For this review, take the finished solid that the model builds, in its own axes (mm). Coordinates: 2 decimals unless noted, no trailing zeros. Loops run counter-clockwise (first coordinate to the right, second up) from the corner with the lowest first, then second, coordinate; pieces in that order, holes last. Notation, with made-up numbers: M 3,21 L 27,21 A14 cw 27,34 Z; hole C 38,-33.75 d11. An arc over 180 degrees is marked long. Answer as a JSON object with one key per item and string values. Group by question number.
Item 1: Insertion check: pin 1 (10 mm diameter, centred on x = -296.88, z = -246.55, fed in from -Y); pin 2 (4 mm diameter, centred on x = -177.8, z = -40.3, fed in from -Y). Each pin has a flat end and moves straight along its axis. Give the tip position at first contact, or say it passes through.
Item 2: Add section A-A (z = -177.8). State the section outline as (x, y) points (3 decimals), then the cut area to 3 significant figures.
Item 3: Add section C-C (y = 1.6). Count the separate pieces of the cut face and the enclosed holes in it, then the cut area to 3 significant figures.
Item 4: Add section B-B (x = -191). State the section outline as (y, z) points (3 decimals), then the cut area to 3 significant figures.
Item 5: Wall thickness on L1, parallel to Z at x = -177.8, y = 1.95 (3 decimals); L2, parallel to X at y = 2.65, z = -316; L3, parallel to X at y = 1.7, z = -246.55: over which ranges is each line inside the solid? List them lowest first. Write a range as from..to.
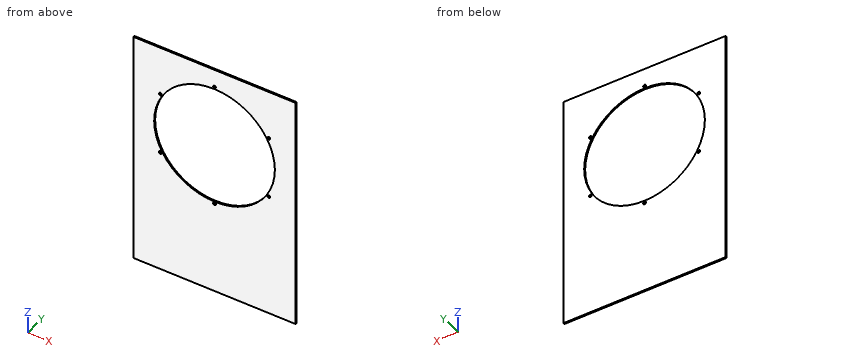
Autodesk Inventor part; units mm, degrees
ref_plane "YZ Plane" through (0, 0, 0) normal (1, 0, 0) x (0, 1, 0)
ref_plane "XZ Plane" through (0, 0, 0) normal (0, 1, 0) x (-1, 0, 0)
ref_plane "XY Plane" through (0, 0, 0) normal (0, 0, 1) x (1, 0, 0)
sketch "Sketch1" plane through (0, 0, 0) normal (0, 1, 0) x (-1, 0, 0)
  line L0 (0, 0) -> (355.6, 0)
  line L1 (355.6, 0) -> (355.6, -520.7)
  line L2 (355.6, -520.7) -> (0, -520.7)
  line L3 (0, -520.7) -> (0, 0)
  circle A0 centre (177.8, -177.8) radius 132.516
  circle A1 centre (177.8, -315.3) radius 3.175
  circle A2 centre (296.8785, -246.55) radius 3.175
  circle A3 centre (296.8785, -109.05) radius 3.175
  circle A4 centre (177.8, -40.3) radius 3.175
  circle A5 centre (58.7215, -109.05) radius 3.175
  circle A6 centre (58.7215, -246.55) radius 3.175
  line L4 (177.8, -177.8) -> (330.2, -177.8) construction
  line L5 (177.8, -177.8) -> (309.7823, -254) construction
  point P0 (177.8, -520.7)
  point P1 (355.6, -260.35)
  dimension "d0" = 355.6
  dimension "d1" = 520.7
  dimension "d2" = 265.032
  dimension "d5" = 177.8
  dimension "d6" = 6.35
  dimension "d7" = 137.5
  dimension "d10" = 360
  dimension "d17" = 152.4
  dimension "d18" = 152.4
  dimension "d19" = 30
  dimension "d22" = 177.8
extrude "Extrusion1" add sketch "Sketch1" along normal blind 3.175
properties part number "TurnTabletBasePlate"
From the geometry:
{
 "1": {"pin 1": "stops at y = 0", "pin 2": "passes through"},
 "2": {"outline": "M -355.6,0 L -310.316,0 L -310.316,3.175 L -355.6,3.175 Z; M -45.284,0 L 0,0 L 0,3.175 L -45.284,3.175 Z", "area": "288 mm²"},
 "3": {"separate pieces": "1", "enclosed holes": "7", "area": "130,000 mm²"},
 "4": {"outline": "M 0,-520.7 L 3.175,-520.7 L 3.175,-309.657 L 0,-309.657 Z; M 0,-45.943 L 3.175,-45.943 L 3.175,0 L 0,0 Z", "area": "816 mm²"},
 "5": {"L1": "z = -520.7..-318.475, -312.125..-310.316, -45.284..-43.475, -37.125..0", "L2": "x = -355.6..-180.9, -174.7..0", "L3": "x = -355.6..-300.05, -293.7..-291.09, -64.51..-61.9, -55.55..0"}
}
